Read the model definition and answer for the solid it produces. Units are mm, in the model's axes. A direction names the side the tool comes from. Coordinates: 2 decimals unless noted, no trailing zeros. Write each loop counter-clockwise with the first axis right and the second up, starting at its lowest first coordinate (ties: lowest second). Pieces come first, ordered by that corner, then holes. Notation, with made-up numbers: (21, -29.5) -> (35, -29.5) arc R25 ccw to (35, 7.5) -> close; hole circle Ø7 at (-1, -3.75). An arc over 180 degrees is marked (long way). One line per item, written item: value. Start each with the question number.
1. Consider line 1 along Y through (x, z) = (44.6, 0); line 2 along X through (y, z) = (-17, 48.5); line 3 along X through (y, z) = (38, 16.5). Determine where each line is inside the solid, lowest interval first.
2. Find section C-C, the plane x = 112. Write down the section's boundary in (y, z), and give its area (3 significant figures).
3. Given P1, Ø5, axis at x = 78.5, y = 17, coming from the -Z side; P2, Ø4, axis at y = -1, z = -42, coming from the -X side; P3, Ø12, axis at y = -38.5, z = -1, coming from the -X side, each flat-ended and moving along its own axis, determine where each tip first touches the part or whether it passes through.
4. For a pull along X with two mould halves and no side action, classify faces 4 (the cylindrical face through (45.47, 8.25, -26.18)), 5 (the cylindrical face through (67.1, -11.59, 15.12)), 6 (the flat face through (46.4, -15, 9)), 7 (the conical face through (48.78, -5.88, -18.67)) as pulls with the +X half, pulls with the -X half, needs draft (parallel to the pull), parting line crosses it, or undercut.
5. Find section B-B, the plane x = 210. Write down the section's boundary in (y, z), and give its area (3 significant figures).
6. For faces 1 (the cylindrical face through (70.16, -5.14, -16.31)), 2 (the cylindrical face through (290.83, 0.315, 7.158)), 3 (the cylindrical face through (55.4, 3.2, -10)), determine the directions among +Z, -Z, +X, -X, +Y, -Y from which every point of the face is accessible in a straight line to the end or side of a thin tool.
7. Find section A-A, the plane x = 52.5. Write down the section's boundary in (y, z).
Autodesk Inventor part; units mm, degrees
ref_plane "YZ Plane" through (0, 0, 0) normal (1, 0, 0) x (0, 1, 0)
ref_plane "XZ Plane" through (0, 0, 0) normal (0, 1, 0) x (-1, 0, 0)
ref_plane "XY Plane" through (0, 0, 0) normal (0, 0, 1) x (1, 0, 0)
sketch "Sketch1" plane through (0, 0, 0) normal (0, 1, 0) x (-1, 0, 0)
  line L0 (0, 0) -> (-303.89, 0)
  line L1 (0, 0) -> (0, -10.5)
  line L2 (0, -10.5) -> (-94.6, -10.5)
  line L3 (-94.6, -10.5) -> (-94.6, -17.1)
  line L4 (-94.6, -17.1) -> (-46.4, -17.1)
  line L5 (-46.4, -17.1) -> (-46.4, -20.31)
  line L6 (-46.4, -20.31) -> (-43.9, -20.31)
  line L7 (-43.9, -20.31) -> (-43.9, -27.45)
  line L8 (-43.9, -27.45) -> (-47, -27.45)
  line L9 (-47, -27.45) -> (-48.9, -19.05)
  line L10 (-48.9, -19.05) -> (-84.8, -19.05)
  line L11 (-84.8, -19.05) -> (-84.8, -37.85)
  line L12 (-84.8, -37.85) -> (-122.9, -37.85)
  line L13 (-122.9, -37.85) -> (-122.9, -25.55)
  line L14 (-122.9, -25.55) -> (-132.9, -40.25)
  line L15 (-132.9, -40.25) -> (-132.9, -40.25)
  line L16 (-132.9, -40.25) -> (-147.9, -40.25)
  line L17 (-147.9, -40.25) -> (-147.9, -46)
  line L18 (-147.9, -46) -> (-150, -46)
  line L19 (-150, -46) -> (-150, -46)
  line L20 (-150, -46) -> (-231.4, -46)
  line L21 (-231.4, -46) -> (-231.4, -56.15)
  line L22 (-231.4, -56.15) -> (-236.2, -56.15)
  line L23 (-236.2, -56.15) -> (-236.2, 0)
  line L24 (-248.9, 0) -> (-248.9, -38.15)
  line L25 (-248.9, -38.15) -> (-277.4, -38.15)
  line L26 (-277.4, -38.15) -> (-277.4, -7.165)
  line L27 (-277.4, -7.165) -> (-303.89, -7.165)
  line L28 (-303.89, -7.165) -> (-303.89, 0)
  line L29 (0, -10.5) -> (0, -12.55)
  line L30 (0, -12.55) -> (-15, -12.55)
  line L31 (-15, -12.55) -> (-15, -10.5)
  line L32 (-236.2, 0) -> (-248.9, 0)
  line L33 (-248.9, 0) -> (-248.9, -30)
  line L34 (-248.9, -30) -> (-236.2, -30)
  line L35 (-236.2, -30) -> (-236.2, 0)
  dimension "d0" = 303.89
  dimension "d1" = 10.5
  dimension "d2" = 94.6
  dimension "d3" = 6.6
  dimension "d4" = 48.2
  dimension "d5" = 3.21
  dimension "d6" = 2.5
  dimension "d7" = 27.45
  dimension "d8" = 3.1
  dimension "d9" = 5
  dimension "d10" = 19.05
  dimension "d11" = 37.8
  dimension "d12" = 37.85
  dimension "d13" = 38.1
  dimension "d14" = 12.3
  dimension "d16" = 10
  dimension "d17" = 40.25
  dimension "d18" = 40.25
  dimension "d19" = 15
  dimension "d20" = 46
  dimension "d21" = 2.1
  dimension "d22" = 46
  dimension "d23" = 98.5
  dimension "d24" = 56.15
  dimension "d25" = 103.3
  dimension "d26" = 12.7
  dimension "d27" = 144.5
  dimension "d28" = 38.15
  dimension "d29" = 90
  dimension "d30" = 7.165
  dimension "d31" = 26.49
  dimension "d54" = 15
  dimension "d55" = 12.55
  dimension "d56" = 30
revolve "Revolution1" add sketch "Sketch1" angle 360 about axis through (0, 0, 0) along (1, 0, 0)
sketch "Sketch6" plane through (236.2, 0, 0) normal (1, 0, 0) x (0, 0, -1)
  line L0 (-25.5477, -44.25) -> (-25.5477, 44.25)
  line L1 (-25.5477, 44.25) -> (51.0955, 0)
  line L2 (51.0955, 0) -> (-25.5477, -44.25)
  circle A0 centre (51.0955, 0) radius 2
  circle A1 centre (-25.5477, -44.25) radius 2
  circle A2 centre (-25.5477, 44.25) radius 2
  point P0 (0, 0)
  point P1 (0, 0)
  dimension "d57" = 4
  dimension "d58" = 88.5
extrude "Extrusion3" cut sketch "Sketch6" against normal up to surface (4.8 mm away) contours L2 A1 L0 | L0 A1 L2 | A2 L1 L0 | L0 L1 A2 | A0 L1 L2 | L2 L1 A0
sketch "Sketch7" plane through (236.2, 0, 0) normal (1, 0, 0) x (0, 0, -1)
  circle A0 centre (0, 0) radius 30
  circle A1 centre (0, 0) radius 41 construction
  circle A2 centre (-29.0395, 28.9432) radius 2.15
  circle A3 centre (-39.9405, 9.2603) radius 2.15
  circle A4 centre (-25.5477, 44.25) radius 2
  dimension "d61" = 11
  dimension "d62" = 4.3
  dimension "d63" = 22.5
  dimension "d64" = 15.7
extrude "Extrusion4" add sketch "Sketch7" along normal blind 15 contours A2 | A3
sketch "Sketch8" plane through (236.2, 0, 0) normal (1, 0, 0) x (0, 0, -1)
  circle A0 centre (0, 0) radius 30
  circle A1 centre (0, 0) radius 40 construction
  circle A2 centre (39.7956, -4.0388) radius 3.05
  circle A3 centre (51.0955, 0) radius 2
  dimension "d67" = 10
  dimension "d68" = 6.1
  dimension "d69" = 12
extrude "Extrusion5" add sketch "Sketch8" along normal blind 61 contours A2
sketch "Sketch9" plane through (297.2, -4.0388, -39.7956) normal (1, 0, 0) x (0, 0, -1)
  circle A0 centre (0, 0) radius 3.05
  circle A1 centre (0, 0) radius 7
  point P0 (-39.7956, 4.0388)
  dimension "d72" = 14
extrude "Extrusion6" add sketch "Sketch9" against normal blind 14 contours A0 | A1
properties part number "STI NGC Cryocooler"
Answer block:
1. line 1: y = -27.45 to -20.31, -10.5 to 10.5, 20.31 to 27.45
1. line 2: x = 231.4 to 236.2
1. line 3: x = 147.9 to 236.2
2. outline: circle Ø75.7 at (0, 0)
2. area: 4,500 mm2
3. P1: stops at z = -12.36
3. P2: stops at x = 132.74
3. P3: stops at x = 84.8
4. face 4: needs draft
4. face 5: undercut
4. face 6: pulls with the -X half
4. face 7: undercut
5. outline: circle Ø92 at (0, 0)
5. area: 6,650 mm2
6. face 1: -X
6. face 2: +X
6. face 3: none
7. outline: circle Ø38.1 at (0, 0); circle Ø21 at (0, 0); hole circle Ø34.2 at (0, 0)
